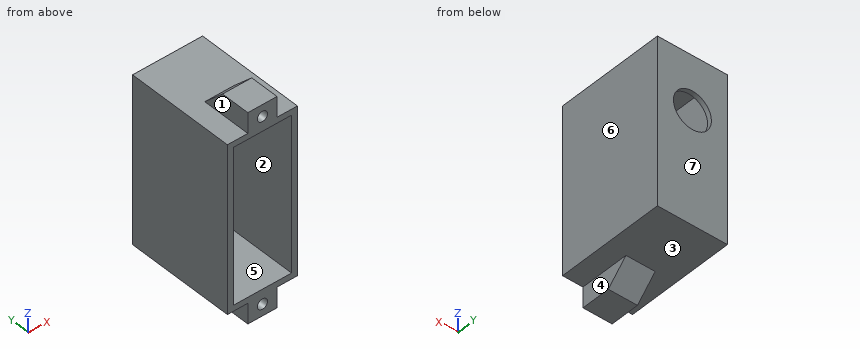
from build123d import *

# Parameters (mm, degrees)
SKETCH1_W           = 20
SKETCH1_H           = 53.2
BOSS_EXTRUDE1_DEPTH = 36
SHELL1_T            = 2
SKETCH2_R           = 6.5
CUT_EXTRUDE1_DEPTH  = 5
SKETCH3_W           = 10
SKETCH3_H           = 10
BOSS_EXTRUDE2_DEPTH = 7
SKETCH4_W           = 10
SKETCH4_H           = 10
BOSS_EXTRUDE3_DEPTH = 7
SKETCH5_R           = 1.75
CUT_EXTRUDE2_DEPTH  = 7
CHAMFER1_SIZE       = 7
SKETCH6_W           = 29.413997259
SKETCH6_H           = 62.11470898
CUT_EXTRUDE3_DEPTH  = 0.5


with BuildPart() as part:
    # Sketch1 → Boss-Extrude1 (new body)
    with BuildSketch(Plane(origin=(0, 0, 0), x_dir=(1, 0, 0), z_dir=(0, 1, 0))):
        Rectangle(SKETCH1_W, SKETCH1_H)
    extrude(amount=BOSS_EXTRUDE1_DEPTH)

    # Shell1
    shell1_openings = [part.faces().sort_by_distance(p)[0] for p in [
        (0, 0, 0),
    ]]
    offset(amount=SHELL1_T, openings=shell1_openings, kind=Kind.INTERSECTION)

    # Sketch2 → Cut-Extrude1 (cut)
    with BuildSketch(Plane(origin=(0, 38, 0), x_dir=(1, 0, 0), z_dir=(0, 1, 0))):
        with Locations(Location((0, -10.1, 0), (0, 0, 270))):
            Circle(SKETCH2_R)
    extrude(amount=-CUT_EXTRUDE1_DEPTH, mode=Mode.SUBTRACT)

    # Sketch3 → Boss-Extrude2 (add)
    with BuildSketch(Plane(origin=(0, 0, -28.6), x_dir=(-1, 0, 0), z_dir=(0, 0, -1))):
        with Locations((0, 5)):
            Rectangle(SKETCH3_W, SKETCH3_H)
    extrude(amount=BOSS_EXTRUDE2_DEPTH)

    # Sketch4 → Boss-Extrude3 (add)
    with BuildSketch(Plane.XY.offset(28.6)):
        with Locations((0, 5)):
            Rectangle(SKETCH4_W, SKETCH4_H)
    extrude(amount=BOSS_EXTRUDE3_DEPTH)

    # Sketch5 → Cut-Extrude2 (cut)
    with BuildSketch(Plane.XZ):
        with Locations(Location((0, 31.6, 0), (0, 0, 270))):
            Circle(SKETCH5_R)
        with Locations(Location((0, -31.6, 0), (0, 0, 270))):
            Circle(SKETCH5_R)
    extrude(amount=-CUT_EXTRUDE2_DEPTH, mode=Mode.SUBTRACT)

    # Chamfer1
    chamfer1_edges = [part.edges().sort_by_distance(p)[0] for p in [
        (0, 10, -28.6),
        (0, 10, 28.6),
    ]]
    chamfer(chamfer1_edges, length=CHAMFER1_SIZE - 0.0001)  # a hair under: the kernel refuses the full size

    # Sketch6 → Cut-Extrude3 (cut)
    with BuildSketch(Plane(origin=(0, 38, 0), x_dir=(1, 0, 0), z_dir=(0, 1, 0))):
        with Locations((0.367646398, -0.2519266)):
            Rectangle(SKETCH6_W, SKETCH6_H)
    extrude(amount=-CUT_EXTRUDE3_DEPTH, mode=Mode.SUBTRACT)


solid = part.part
The listing builds one solid part. Answer for the finished solid, in the listing's coordinates (mm). Face numbers are marked on the shaded views. A direction names the side the tool comes from. Coordinates: 2 decimals unless noted, no trailing zeros. Write each loop counter-clockwise with the first axis right and the second up, starting at its lowest first coordinate (ties: lowest second). Pieces come first, ordered by that corner, then holes. Notation, with made-up numbers: (80.5, -39) - (85.5, -39) arc R18 ccw to (85.5, -21) - close; hole circle Ø7 at (58.25, 77.25). An arc over 180 degrees is marked (long way). Put each result on its own line as item: value.
1. The part is cut by section C-C on z = -1. Give the vertices of the cut face in (x, y).
Answer sheet:
outline: (-12, 0) - (-10, 0) - (-10, 36) - (10, 36) - (10, 0) - (12, 0) - (12, 37.5) - (-12, 37.5) - close
2. The part is cut by section A-A on y = 30. Give the vertices of the cut face in (x, z).
Answer sheet:
outline: (-12, -28.6) - (12, -28.6) - (12, 28.6) - (-12, 28.6) - close; hole (-10, -26.6) - (10, -26.6) - (10, 26.6) - (-10, 26.6) - close
3. The part is cut by section D-D on x = 9. Give the vertices of the cut face in (y, z), plus the area to 3 significant figures.
Answer sheet:
outline: (0, -28.6) - (37.5, -28.6) - (37.5, 28.6) - (0, 28.6) - (0, 26.6) - (36, 26.6) - (36, -26.6) - (0, -26.6) - close
area: 230 mm^2
4. Flat-ended cylindrical pins translate along their axes: pin 1 Ø10 at (x, z) = (-2.5, -6.5) entering from -Y; pin 2 Ø12 at (x, y) = (-0.5, 23.5) entering from -Z; pin 3 Ø1 at (x, z) = (0.5, 31) entering from -Y. Find the tip coordinate at first contact, or state that the pin passes through.
Answer sheet:
pin 1: stops at y = 36
pin 2: stops at z = -28.6
pin 3: stops at y = 7
5. A tool of negligible diameter and unlimited length cuts with its end or side. For the marked faces 1, 2, 3 and 4, from which of +Z, -Z, +X, -X, +Y, -Y can it reach the whole face along a straight path? Write none if from no direction.
Answer sheet:
face 1: +Z, -X, +Y, -Y
face 2: -Y
face 3: -Z, +Y
face 4: -Z, +X, +Y, -Y
6. Find the intervals of material crossed by line 1 along X through (y, z) = (3, 31.6); line 2 along X through (y, z) = (14, -19); line 3 along Z through (x, y) = (1.25, 29.5), in increasing order. Write a range as from..to.
Answer sheet:
line 1: x = -5..-1.75, 1.75..5
line 2: x = -12..-10, 10..12
line 3: z = -28.6..-26.6, 26.6..28.6
7. Determine the mould class of the marked faces 5, 6 and 7 for opening direction X: pulls with the +X half, pulls with the -X half, needs draft (parallel to the pull), parting line crosses it, or undercut.
Answer sheet:
face 5: undercut
face 6: pulls with the +X half
face 7: needs draft
